Read the model definition and answer for the solid it produces. Units are mm, in the model's axes. A direction names the side the tool comes from. Coordinates: 2 decimals unless noted, no trailing zeros. Loops run counter-clockwise (first coordinate to the right, second up) from the corner with the lowest first, then second, coordinate; pieces in that order, holes last.
from build123d import *

# Parameters (mm, degrees)
F0_W     = 42.418
F0_H     = 33.02
F1_DEPTH = 4.6228
F2_W     = 42.418
F2_H     = 10.7696
F3_DEPTH = 9.525
F4_R     = 2.9718
F5_DEPTH = 50.8


with BuildPart() as f1:
    # F0 (on Top) → F1 (new body)
    with BuildSketch(Plane.XY):
        Rectangle(F0_W, F0_H)
    extrude(amount=F1_DEPTH)

    # F2 (on face) → F3 (join)
    with BuildSketch(Plane.XY.offset(4.6228)):
        Rectangle(F2_W, F2_H)
    extrude(amount=F3_DEPTH)

    # F4 (on face) → F5 (cut)
    with BuildSketch(Plane.YZ.offset(21.209)):
        with Locations((0, 6.6548)):
            Circle(F4_R)
    extrude(amount=-F5_DEPTH, mode=Mode.SUBTRACT)


solid = f1.part
Q1. A cutting plane is placed at B-B (z = 9). Give the vertices of the cut face in (x, y).
Findings below:
outline: (-21.21, -5.38) - (21.21, -5.38) - (21.21, -1.83) - (-21.21, -1.83) - close; (-21.21, 1.83) - (21.21, 1.83) - (21.21, 5.38) - (-21.21, 5.38) - close
Q2. Straight lines are drawn through the part: probe 1 along Z at (x, y) = (1.5, 0); probe 2 along Z at (x, y) = (-3, -6); probe 3 along Z at (x, y) = (3, 2.5). For each, find the intervals that lie inside material, in ascending order.
Findings below:
probe 1: z = 0 to 3.68, 9.63 to 14.15
probe 2: z = 0 to 4.62
probe 3: z = 0 to 5.05, 8.26 to 14.15
Q3. Determine the mould class of faces 4 (the face through (0, -16.51, 2)), 5 (the face through (0, 0, 14.148)), 6 (the face through (0.297, -0.644, 3.754)), 7 (the face through (0, 5.385, 9)) for opening direction Y: +Y half, -Y half, draft (parallel to the pull), parting line (faces both ways), or undercut.
Findings below:
face 4: -Y half
face 5: draft
face 6: undercut
face 7: +Y half
Q4. Flat-ended cylindrical pins translate along their axes: pin 1 Ø3 at (x, z) = (-7.5, 9.5) entering from +Y; pin 2 Ø3 at (x, z) = (1, 8.5) entering from -Y; pin 3 Ø5.5 at (x, y) = (-1, -9.5) entering from +Z. Find the tip coordinate at first contact, or state that the pin passes through.
Findings below:
pin 1: stops at y = 5.38
pin 2: stops at y = -5.38
pin 3: stops at z = 4.62
Q5. A cutting plane is placed at A-A (y = 0). Give the vertices of the cut face in (x, z), then the cut area to 3 significant figures.
Findings below:
outline: (-21.21, 0) - (21.21, 0) - (21.21, 3.68) - (-21.21, 3.68) - close; (-21.21, 9.63) - (21.21, 9.63) - (21.21, 14.15) - (-21.21, 14.15) - close
area: 348 mm2
Q6. A cutting plane is placed at D-D (y = 13). Give the vertices of the cut face in (x, z).
Findings below:
outline: (-21.21, 0) - (21.21, 0) - (21.21, 4.62) - (-21.21, 4.62) - close
Q7. A cutting plane is placed at C-C (x = 16.5). Give the vertices of the cut face in (y, z).
Findings below:
outline: (-16.51, 0) - (16.51, 0) - (16.51, 4.62) - (5.38, 4.62) - (5.38, 14.15) - (-5.38, 14.15) - (-5.38, 4.62) - (-16.51, 4.62) - close; hole circle Ø5.94 at (0, 6.65)
Q8. Which of the six approach directions +Z, -Z, +X, -X, +Y, -Y give full straight-line access (tool end or side, diameter ignored) to faces 1 (the face through (0, -11, 4.623)), 2 (the face through (0, 11, 4.623)), 3 (the face through (0, 16.51, 2))?
Findings below:
face 1: +Z, +X, -X, -Y
face 2: +Z, +X, -X, +Y
face 3: +Z, -Z, +X, -X, +Y
